Here's the drawing with two shaded views (mm, measured from the low corner). I have some questions. Give positions to 0.01 mm unless a question says otherwise; leave off trailing zeros. Loops run counter-clockwise (first coordinate to the right, second up) from the corner with the lowest first, then second, coordinate; pieces in that order, holes last. Notation, with made-up numbers: M -8.75,79 L 39.25,79 A30 cw 39.25,105 Z; hole C 42,30 d5. An arc over 180 degrees is marked long. Use CSV: the item, a comma, the result in double quotes.
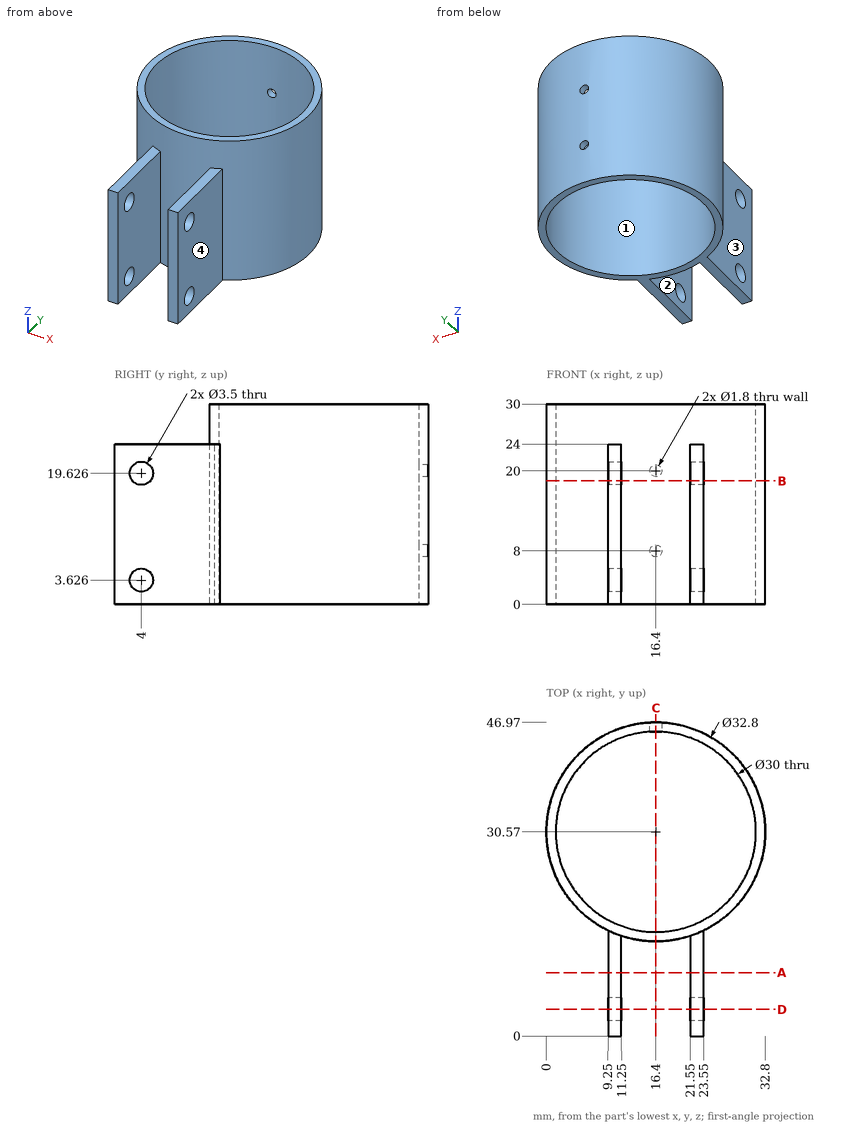
1. I want a section at B-B, the plane z = 18.5. List the corners of the cut face in (x, y) for me.
Outcome:
outline,"M 9.25,0 L 11.25,0 L 11.25,2.66 L 9.25,2.66 Z; M 9.25,5.34 L 11.25,5.34 L 11.25,15 A16.4 ccw 21.55,15 L 21.55,5.34 L 23.55,5.34 L 23.55,15.81 A16.4 ccw long 9.25,15.81 Z; M 21.55,0 L 23.55,0 L 23.55,2.66 L 21.55,2.66 Z; hole C 16.4,30.57 d30"
2. If we mould it in two halves opening along X, with no side actions, what happens to the marked faces 1, 2, 3 and 4? For each: +X half, -X half, draft (parallel to the pull), parting line (faces both ways), or undercut.
Outcome:
face 1,"undercut"
face 2,"undercut"
face 3,"-X half"
face 4,"+X half"
3. I'm going to push flat-ended pins straight in: pin 1 Ø6 at (y, z) = (41.5, 24.5) entering from -X (1 decimal); pin 2 Ø7.5 at (y, z) = (10.5, 14.5) entering from -X; pin 3 Ø1.6 at (x, z) = (16.4, 20) entering from -Y. Where does each tip first touch, or does it pass through?
Outcome:
pin 1,"x = 2"
pin 2,"x = 9.25"
pin 3,"y = 14.17"
4. I want a section at D-D, the plane y = 4. List the corners of the cut face in (x, z) for me.
Outcome:
outline,"M 9.25,0 L 11.25,0 L 11.25,1.88 L 9.25,1.88 Z; M 9.25,5.38 L 11.25,5.38 L 11.25,17.88 L 9.25,17.88 Z; M 9.25,21.38 L 11.25,21.38 L 11.25,24 L 9.25,24 Z; M 21.55,0 L 23.55,0 L 23.55,1.88 L 21.55,1.88 Z; M 21.55,5.38 L 23.55,5.38 L 23.55,17.88 L 21.55,17.88 Z; M 21.55,21.38 L 23.55,21.38 L 23.55,24 L 21.55,24 Z"
5. Please list where these lines run through material, in increasing order: line 1 (Z direction, x = 16.4, y = 46.25); line 2 (X direction, y = 12.5, z = 4); line 3 (Z direction, x = 16, y = 46) (1 decimal).
Outcome:
line 1,"0 to 7.1, 8.9 to 19.1, 20.9 to 30"
line 2,"9.25 to 11.25, 21.55 to 23.55"
line 3,"0 to 7.2, 8.8 to 19.2, 20.8 to 30"
6. I want a section at A-A, the plane y = 9.5. List the corners of the cut face in (x, z) for me.
Outcome:
outline,"M 9.25,0 L 11.25,0 L 11.25,24 L 9.25,24 Z; M 21.55,0 L 23.55,0 L 23.55,24 L 21.55,24 Z"
7. I want a section at C-C, the plane x = 16.4. List the corners of the cut face in (y, z) for me.
Outcome:
outline,"M 14.17,0 L 15.57,0 L 15.57,30 L 14.17,30 Z; M 45.57,0 L 46.97,0 L 46.97,7.1 L 45.57,7.1 Z; M 45.57,8.9 L 46.97,8.9 L 46.97,19.1 L 45.57,19.1 Z; M 45.57,20.9 L 46.97,20.9 L 46.97,30 L 45.57,30 Z"
